Could you check a few things on this model? Use its own coordinates, in mm. A direction names the side the tool comes from. Round coordinates to 2 decimals unless told otherwise and drop trailing zeros. Write each loop counter-clockwise with the first axis right and the second up, starting at its lowest first coordinate (ties: lowest second). Pieces come first, ordered by that corner, then holes. Notation, with made-up numbers: (15.5, 23.5) -> (64.5, 23.5) arc R32 cw to (64.5, 54.5) -> close; hole circle Ø7 at (-14, 0). An arc over 180 degrees is marked (long way). Return JSON: item names as keys, results as strings.
from build123d import *

# Parameters (mm, degrees)
SKETCH1_W           = 622.3
SKETCH1_H           = 419.1
BOSS_EXTRUDE1_DEPTH = 107.95
SKETCH4_R           = 30.1625
CUT_EXTRUDE3_DEPTH  = 108.95
SKETCH5_W           = 381
SKETCH5_H           = 228.6
CUT_EXTRUDE4_DEPTH  = 6.35


with BuildPart() as part:
    # Sketch1 → Boss-Extrude1 (new body)
    with BuildSketch(Plane(origin=(0, 0, 0), x_dir=(1, 0, 0), z_dir=(0, 1, 0))):
        Rectangle(SKETCH1_W, SKETCH1_H)
    extrude(amount=BOSS_EXTRUDE1_DEPTH)

    # Sketch4 → Cut-Extrude3 (cut, through all)
    with BuildSketch(Plane(origin=(0, 107.95, 0), x_dir=(1, 0, 0), z_dir=(0, 1, 0))):
        with Locations((-114.3, 68.58)):
            Circle(SKETCH4_R)
        with Locations((-114.3, -68.58)):
            Circle(SKETCH4_R)
        with Locations((114.3, 68.58)):
            Circle(SKETCH4_R)
        with Locations((114.3, -68.58)):
            Circle(SKETCH4_R)
    extrude(amount=-CUT_EXTRUDE3_DEPTH, mode=Mode.SUBTRACT)

    # Sketch5 → Cut-Extrude4 (cut)
    with BuildSketch(Plane(origin=(0, 107.95, 0), x_dir=(1, 0, 0), z_dir=(0, 1, 0))):
        Rectangle(SKETCH5_W, SKETCH5_H)
    extrude(amount=-CUT_EXTRUDE4_DEPTH, mode=Mode.SUBTRACT)


solid = part.part
1) I want a section at A-A, the plane z = 68.58. Please give me the cut outline in (x, y).
Return value:
{"outline": "(-311.15, 0) -> (-144.46, 0) -> (-144.46, 101.6) -> (-190.5, 101.6) -> (-190.5, 107.95) -> (-311.15, 107.95) -> close; (-84.14, 0) -> (84.14, 0) -> (84.14, 101.6) -> (-84.14, 101.6) -> close; (144.46, 0) -> (311.15, 0) -> (311.15, 107.95) -> (190.5, 107.95) -> (190.5, 101.6) -> (144.46, 101.6) -> close"}
2) I want a section at C-C, the plane y = 8. Count the separate pieces of the cut face and the enclosed holes in it, and give its area (3 significant figures).
Return value:
{"separate pieces": "1", "enclosed holes": "4", "area": "249,000 mm²"}
3) I want a section at D-D, the plane z = 2.5. Please give me the cut outline in (x, y).
Return value:
{"outline": "(-311.15, 0) -> (311.15, 0) -> (311.15, 107.95) -> (190.5, 107.95) -> (190.5, 101.6) -> (-190.5, 101.6) -> (-190.5, 107.95) -> (-311.15, 107.95) -> close"}
4) Will this pin go through, and if not, where does the flat tip stop? pin 1 Ø6 at (x, z) = (-61.5, -156.5) entering from -Y.
Return value:
{"pin 1": "y = 0"}
5) I want a section at B-B, the plane x = 114.3. Please give me the cut outline in (y, z).
Return value:
{"outline": "(0, -209.55) -> (107.95, -209.55) -> (107.95, -114.3) -> (101.6, -114.3) -> (101.6, -98.74) -> (0, -98.74) -> close; (0, -38.42) -> (101.6, -38.42) -> (101.6, 38.42) -> (0, 38.42) -> close; (0, 98.74) -> (101.6, 98.74) -> (101.6, 114.3) -> (107.95, 114.3) -> (107.95, 209.55) -> (0, 209.55) -> close"}
6) For faces 4 (the face through (-3, 101.6, -2)), 5 (the face through (-311.15, 53, 3)), which set-ups out of +Z, -Z, +X, -X, +Y, -Y let a thin tool reach every point of the face, with its end or its side?
Return value:
{"face 4": "+Y", "face 5": "+Z, -Z, -X, +Y, -Y"}
7) Thinking about a two-plate mould opening in Z: for faces 1 (the face through (130.52, 51.51, 43.15)), 2 (the face through (-4, 107.95, 137)), 3 (the face through (-4, 53, 209.55)), which applies, pulls with the +Z half, pulls with the -Z half, needs draft (parallel to the pull), parting line crosses it, or undercut?
Return value:
{"face 1": "undercut", "face 2": "needs draft", "face 3": "pulls with the +Z half"}
8) If I drill on probe 1 along X at (y, z) = (86, 68.5); probe 2 along Z at (x, y) = (114.3, 35); probe 3 along X at (y, z) = (66.5, 92.5), over which ranges is the centre line in solid material (lowest first)? Write a range as [from, to].
Return value:
{"probe 1": "[-311.15, -144.46], [-84.14, 84.14], [144.46, 311.15]", "probe 2": "[-209.55, -98.74], [-38.42, 38.42], [98.74, 209.55]", "probe 3": "[-311.15, -132.67], [-95.93, 95.93], [132.67, 311.15]"}
